Autodesk Inventor part; units mm, degrees
ref_plane "YZ Plane" through (0, 0, 0) normal (1, 0, 0) x (0, 1, 0)
ref_plane "XZ Plane" through (0, 0, 0) normal (0, 1, 0) x (-1, 0, 0)
ref_plane "XY Plane" through (0, 0, 0) normal (0, 0, 1) x (1, 0, 0)
sketch "Boceto4" plane through (0, 0, 0) normal (0, 0, 1) x (1, 0, 0)
  circle A0 centre (-1.0562, 12.2493) radius 5
  line L0 (33.4438, -22.7507) -> (-36.5562, -22.7507)
  line L1 (33.4438, 47.2493) -> (33.4438, -22.7507)
  line L2 (-36.5562, 47.2493) -> (33.4438, 47.2493)
  line L3 (-36.5562, -22.7507) -> (-36.5562, 47.2493)
  circle A1 centre (21.3438, 12.2493) radius 3.7
  circle A2 centre (-23.4562, 12.2493) radius 3.7
  line L4 (36.4438, 50.2493) -> (-39.5562, 50.2493)
  line L5 (-39.5562, 50.2493) -> (-39.5562, -25.7507)
  line L6 (-39.5562, -25.7507) -> (36.4438, -25.7507)
  line L7 (36.4438, -25.7507) -> (36.4438, 50.2493)
  line L8 (33.4438, -22.7507) -> (-36.5562, -22.7507)
  line L9 (-36.5562, -22.7507) -> (-36.5562, 47.2493)
  line L10 (-36.5562, 47.2493) -> (33.4438, 47.2493)
  line L11 (33.4438, 47.2493) -> (33.4438, -22.7507)
  point P0 (0, 0)
extrude "Extrusión4" add sketch "Boceto4" against normal blind 10 contours L7 L6 L5 L4
sketch "Boceto5" plane through (0, 0, 0) normal (0, 0, 1) x (1, 0, 0)
  line L0 (-39.5562, 50.2493) -> (-39.5562, -25.7507)
  line L1 (-39.5562, -25.7507) -> (36.4438, -25.7507)
  line L2 (36.4438, -25.7507) -> (36.4438, 50.2493)
  line L3 (36.4438, 50.2493) -> (-39.5562, 50.2493)
  line L4 (-36.5562, -22.7507) -> (-36.5562, 47.2493)
  line L5 (-36.5562, 47.2493) -> (33.4438, 47.2493)
  line L6 (33.4438, 47.2493) -> (33.4438, -22.7507)
  line L7 (33.4438, -22.7507) -> (-36.5562, -22.7507)
  circle A0 centre (-1.0562, 12.2493) radius 5
  line L8 (33.4438, -22.7507) -> (-36.5562, -22.7507)
  line L9 (33.4438, 47.2493) -> (33.4438, -22.7507)
  line L10 (-36.5562, 47.2493) -> (33.4438, 47.2493)
  line L11 (-36.5562, -22.7507) -> (-36.5562, 47.2493)
  circle A1 centre (21.3438, 12.2493) radius 3.7
  circle A2 centre (-23.4562, 12.2493) radius 3.7
  point P0 (0, 0)
extrude "Extrusión5" add sketch "Boceto5" along normal blind 2 contours L3 L2 L1 L0 | L4 L5 L6 L7
sketch "Boceto6" plane through (0, 0, 0) normal (0, 0, -1) x (-1, 0, 0)
  line L0 (39.5562, 50.2493) -> (-36.4438, 50.2493)
  line L1 (-36.4438, 50.2493) -> (-36.4438, -25.7507)
  line L2 (-36.4438, -25.7507) -> (39.5562, -25.7507)
  line L3 (39.5562, -25.7507) -> (39.5562, 50.2493)
  circle A0 centre (1.0562, 12.2493) radius 5
  circle A1 centre (-21.3438, 12.2493) radius 3.7
  circle A2 centre (23.4562, 12.2493) radius 3.7
  circle A3 centre (5.2662, -1.7699) radius 1.5
  circle A4 centre (-7.7338, -1.7699) radius 1.5
  point P0 (0, 0)
extrude "Extrusión6" add sketch "Boceto6" against normal blind 2 contours A0 | A1 | A2
sketch "Boceto8" plane through (0, 0, 0) normal (0, 0, -1) x (-1, 0, 0)
  circle A0 centre (5.2662, -1.7699) radius 1.5
  circle A1 centre (-7.7338, -1.7699) radius 1.5
  point P0 (0, 0)
extrude "Extrusión7" cut sketch "Boceto8" against normal blind 2
properties part number "sensor_estructura"
Geometry: final body of the model. Coordinates: model frame, mm. A direction names the side the tool comes from. Round coordinates to 2 decimals unless told otherwise and drop trailing zeros. Write each loop counter-clockwise with the first axis right and the second up, starting at its lowest first coordinate (ties: lowest second). Pieces come first, ordered by that corner, then holes.
Item 1: Set-up query: faces 4 (the face through (-2, 13, 2)), 5 (the face through (-1, -22.751, -5)). Return all of +Z, -Z, +X, -X, +Y, -Y with unobstructed straight access to the full face (end or side cutting, diameter ignored); none if empty.
Item 2: Section query C-C (x = 31). Return loops of the section in (y, z).
Item 3: Material intervals for L1, parallel to Y at x = -21, z = -7.5; L2, parallel to X at y = 15, z = -5.5; L3, parallel to Z at x = 30, y = 17, sorted ascending.
Item 4: Pin query (flat end, axial travel): P1, Ø1.5, axis at x = 5.5, y = -16, coming from the -Z side. Return the tip coordinate at first contact, or that it passes through.
Item 5: Mould query, pull axis Y, two halves, no side actions, for faces 1 (the face through (-2, -25.751, -4)), 2 (the face through (-2, 47.249, -5)), 3 (the face through (-1, 50.249, -4)). Classes: +Y half, -Y half, draft (parallel to the pull), parting line (faces both ways), or undercut.
Item 6: Section query B-B (y = 40.5). Return loops of the section in (x, z).
Item 7: Section query A-A (z = -1). Return loops of the section in (x, y).
Completed:
1. face 4: +Z, +X, -X, +Y, -Y
1. face 5: -Z
2. outline: (-25.75, -10) - (-22.75, -10) - (-22.75, 0) - (47.25, 0) - (47.25, -10) - (50.25, -10) - (50.25, 2) - (-25.75, 2) - close
3. L1: y = -25.75 to -22.75, 47.25 to 50.25
3. L2: x = -39.56 to -36.56, 33.44 to 36.44
3. L3: z = 0 to 2
4. P1: stops at z = 0
5. face 1: -Y half
5. face 2: undercut
5. face 3: +Y half
6. outline: (-39.56, -10) - (-36.56, -10) - (-36.56, 0) - (33.44, 0) - (33.44, -10) - (36.44, -10) - (36.44, 2) - (-39.56, 2) - close
7. outline: (-39.56, -25.75) - (36.44, -25.75) - (36.44, 50.25) - (-39.56, 50.25) - close; hole (-36.56, -22.75) - (33.44, -22.75) - (33.44, 47.25) - (-36.56, 47.25) - close
